Read the model definition and answer for the solid it produces. Units are mm, in the model's axes. Give positions to 0.01 mm unless a question says otherwise; leave off trailing zeros. Write each loop counter-clockwise with the first axis right and the second up, starting at its lowest first coordinate (ties: lowest second). Pieces come first, ordered by that corner, then holes. Notation, with made-up numbers: (20.5, -13.75) -> (47.5, -13.75) arc R24 cw to (47.5, 23.25) -> close; hole circle Ø9 at (3, 71). An arc over 180 degrees is marked (long way). Use a Markdown table: item, result.
Autodesk Fusion 360 part; units mm, degrees
sketch "Sketch1" plane through (0, 0, 0) normal (0, 0, 1) x (1, 0, 0)
  circle A0 centre (8.6658, 10.0855) radius 1.15
  dimension "d1" = 2.3
extrude "Extrude1" add sketch "Sketch1" along normal blind 120
extrude "Extrude2" cut 1 faces at (8.9089, 10.1799, 120) along direction (0, 0, -1) blind 20
chamfer "Chamfer1" distance 0.5 angle 45 2 faces at (8.9089, 10.1799, 100) (9.7701, 9.7644, 33.3333)
Item 1: Each of these flat-tipped pins is pushed along its axis until it touches: P1, Ø1, axis at x = 9.5, y = 10.5, coming from the +Z side; P2, Ø1, axis at x = 9.5, z = 55.5, coming from the +Y side. Where does it stop, or does it pass through?
Return value:
| item | result |
|---|---|
| P1 | z = 100 |
| P2 | y = 11.19 |
Item 2: Straight lines are drawn through the part: line 1 along Z through (x, y) = (8, 10.1); line 2 along X through (y, z) = (9.9, 21); line 3 along Y through (x, z) = (8.85, 84.5). For each, find the intervals that lie inside material, in ascending order. Write a range as [from, to].
Return value:
| item | result |
|---|---|
| line 1 | [0.02, 99.98] |
| line 2 | [7.53, 9.8] |
| line 3 | [8.95, 11.22] |
Item 3: A cutting plane is placed at A-A (z = 42.5). Give the vertices of the cut face in (x, y), then the cut area to 3 significant figures.
Return value:
| item | result |
|---|---|
| outline | circle Ø2.3 at (8.67, 10.09) |
| area | 4.15 mm^2 |
